The listing builds one solid part. Answer for the finished solid, in the listing's coordinates (mm). Face numbers are marked on the shaded views. A direction names the side the tool comes from. Give positions to 0.01 mm unless a question says otherwise; leave off trailing zeros. Loops run counter-clockwise (first coordinate to the right, second up) from the corner with the lowest first, then second, coordinate; pieces in that order, holes last. Notation, with made-up numbers: (37, -13) - (83, -13) arc R18 ccw to (83, -9) - close; hole circle Ø10 at (-27, 81.25). An arc over 180 degrees is marked (long way). Write each question's results on one line, items separated by ' | '.
from build123d import *

# Parameters (mm, degrees)
F0_R     = 1.524
F1_DEPTH = 1.905
F2_R     = 0.3175
F3_DEPTH = 25.4
F4_R     = 5.08
F5_DEPTH = 3.83728


with BuildPart() as f1:
    # F0 (on Front) → F1 (new body)
    with BuildSketch(Plane.XZ):
        with BuildLine():
            ThreePointArc((0, -5.08), (3.592102, -3.592102), (5.08, 0))
            ThreePointArc((5.08, 0), (3.592102, 3.592102), (0, 5.08))
            Line((0, 5.08), (0, -5.08))
        make_face()
        with BuildLine():
            ThreePointArc((0, -5.08), (-5.08, 0), (0, 5.08))
            Line((0, 5.08), (-33.02, 5.08))
            Line((-33.02, 5.08), (-33.02, -5.08))
            Line((-33.02, -5.08), (0, -5.08))
        make_face()
        with Locations((-17.78, 0)):
            Circle(F0_R, mode=Mode.SUBTRACT)
    extrude(amount=F1_DEPTH)

    # F2 (on face) → F3 (join)
    with BuildSketch(Plane(origin=(0, 0, -5.08), x_dir=(1, 0, 0), z_dir=(0, 0, -1))):
        with Locations((-31.115, 1.9304)):
            Circle(F2_R)
        with Locations((-28.575, 1.9304)):
            Circle(F2_R)
        with Locations((-26.035, 1.9304)):
            Circle(F2_R)
        with Locations((-23.495, 1.9304)):
            Circle(F2_R)
    extrude(amount=F3_DEPTH)

    # F4 (on face) → F5 (cut)
    with BuildSketch(Plane(origin=(0, 0, 0), x_dir=(-1, 0, 0), z_dir=(0, 1, 0))):
        Circle(F4_R)
    extrude(amount=-F5_DEPTH, mode=Mode.SUBTRACT)


solid = f1.part
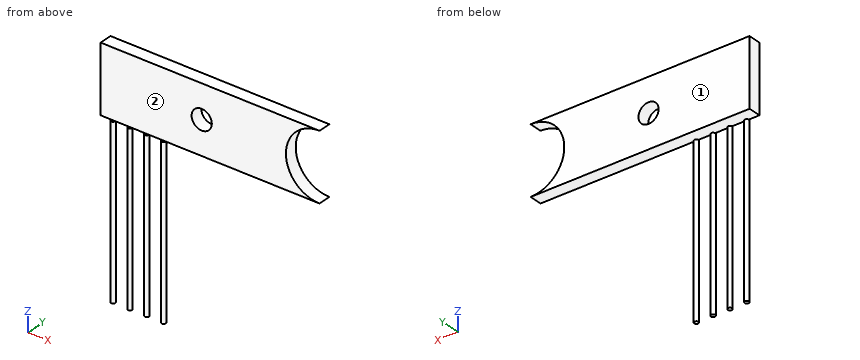
Item 1: Find the intervals of material crossed by line 1 along Z through (x, y) = (-17.78, -1.2); line 2 along X through (y, z) = (-1.9, -7.5); line 3 along Z through (x, y) = (-25.5, -1.7), in increasing order. Write a range as [from, to].
Values found:
line 1: z = [-5.08, -1.52], [1.52, 5.08] | line 2: x = [-31.43, -30.8], [-28.89, -28.26], [-26.35, -25.72], [-23.81, -23.18] | line 3: z = [-5.08, 5.08]
Item 2: For the marked faces 1 and 2, determine the directions among +Z, -Z, +X, -X, +Y, -Y from which every point of the face is accessible in a straight line to the end or side of a thin tool.
Values found:
face 1: +Z, -Z, +X, -X, +Y | face 2: +Z, +X, -X, -Y
Item 3: Flat-ended cylindrical pins translate along their axes: P1, Ø3, axis at x = -17, z = -2, coming from the -Y side (3 decimals); P2, Ø1, axis at x = -9, y = -1, coming from the -Z side. Find the tip coordinate at first contact, or state that the pin passes through.
Values found:
P1: stops at y = -1.905 | P2: stops at z = -5.08
Item 4: A cutting plane is placed at D-D, the plane x = -21.5. Determine the outline of the cut face in (y, z) (3 decimals).
Values found:
outline: (-1.905, -5.08) - (0, -5.08) - (0, 5.08) - (-1.905, 5.08) - close
Item 5: A cutting plane is placed at C-C, the plane y = -1. Determine the outline of the cut face in (x, z), plus the area to 3 significant figures.
Values found:
outline: (-33.02, -5.08) - (0, -5.08) arc R5.08 cw to (0, 5.08) - (-33.02, 5.08) - close; hole circle Ø3.05 at (-17.78, 0) | area: 288 mm²
Item 6: A cutting plane is placed at A-A, the plane x = -17.78. Determine the outline of the cut face in (y, z) (3 decimals).
Values found:
outline: (-1.905, -5.08) - (0, -5.08) - (0, -1.524) - (-1.905, -1.524) - close; (-1.905, 1.524) - (0, 1.524) - (0, 5.08) - (-1.905, 5.08) - close
Item 7: A cutting plane is placed at B-B, the plane z = 0. Determine the outline of the cut face in (x, y) (3 decimals).
Values found:
outline: (-33.02, -1.905) - (-19.304, -1.905) - (-19.304, 0) - (-33.02, 0) - close; (-16.256, -1.905) - (-5.08, -1.905) - (-5.08, 0) - (-16.256, 0) - close
